Source: CAD feature listing. Evaluate the final solid. Frame: model axes, mm. Coordinates: 2 decimals unless noted, no trailing zeros. Write each loop counter-clockwise with the first axis right and the second up, starting at its lowest first coordinate (ties: lowest second). Pieces come first, ordered by that corner, then holes. Notation, with made-up numbers: (83.5, 33.25) -> (100.5, 33.25) arc R34 ccw to (100.5, 72.25) -> close; hole circle Ø3 at (85.5, -11.75). An arc over 180 degrees is marked (long way). Write item = value, one per line.
Solid Edge part; units mm, degrees
sketch "Sketch1" plane through (0, 0, 0) normal (0, 0, 1) x (1, 0, 0)
  circle A0 centre (0, 0) radius 1
extrude "Protrusion1" add sketch "Sketch1" along normal blind 10
sketch "Sketch2" plane through (0, 0, 10) normal (0, 0, 1) x (1, 0, 0)
  circle A0 centre (0, 0) radius 2
extrude "ProtrusiónExtruida_2" add sketch "Sketch2" along normal blind 0.2
chamfer "Chaflán_2" distance 1 angle 45 1 edges at (1, 0, 10)
sketch "Sketch3" plane through (0, 0, 10.2) normal (0, 0, 1) x (1, 0, 0)
  line L0 (0, -1) -> (-0.3536, -0.3536)
  line L1 (-0.3536, -0.3536) -> (-1, 0)
  line L2 (-1, 0) -> (-0.3536, 0.3536)
  line L3 (-0.3536, 0.3536) -> (0, 1)
  line L4 (0, 1) -> (0.3536, 0.3536)
  line L5 (0.3536, 0.3536) -> (1, 0)
  line L6 (1, 0) -> (0.3898, -0.3898)
  line L7 (0.3898, -0.3898) -> (0, -1)
extrude "VaciadoExtruido_1" cut sketch "Sketch3" against normal blind 0.5
chamfer "Chaflán_1" distance 1 angle 45 1 edges at (-1, 0, 0)
properties material "Latón, amarillo"
1) Pull-direction query (Y, two-part tool) for faces 1 (the cylindrical face through (0, 1, 5)), 2 (the flat face through (0, 0, 9.7)), 3 (the flat face through (-0.5, 0.5, 10.2)); classes: +Y half, -Y half, draft (parallel to the pull), parting line (faces both ways), or undercut.
Answer block:
face_1 = parting line
face_2 = undercut
face_3 = draft
2) Material intervals for probe 1 along X at (y, z) = (-0.05, 1.5); probe 2 along Z at (x, y) = (1.4, -0.05), sorted ascending. Write a range as [from, to].
Answer block:
probe_1 = [-1, 1]
probe_2 = [9.4, 10.2]
3) First-contact query: pin 1 Ø1 at (x, y) = (-1.5, -1) entering from -Z; pin 2 Ø1.5 at (y, z) = (-1.5, 6) entering from -X; pin 3 Ø1.5 at (y, z) = (0, 7.5) entering from +X. Flat tips, straight axial feed; report the tip coordinate or a pass-through.
Answer block:
pin_1 = 9.3
pin_2 = -0.66
pin_3 = 1
4) Cut plane A-A, the plane z = 2.5. Output: boundary loops of the cut face in (x, y), and give its area (3 significant figures).
Answer block:
outline = circle Ø2 at (0, 0)
area = 3.14 mm2
